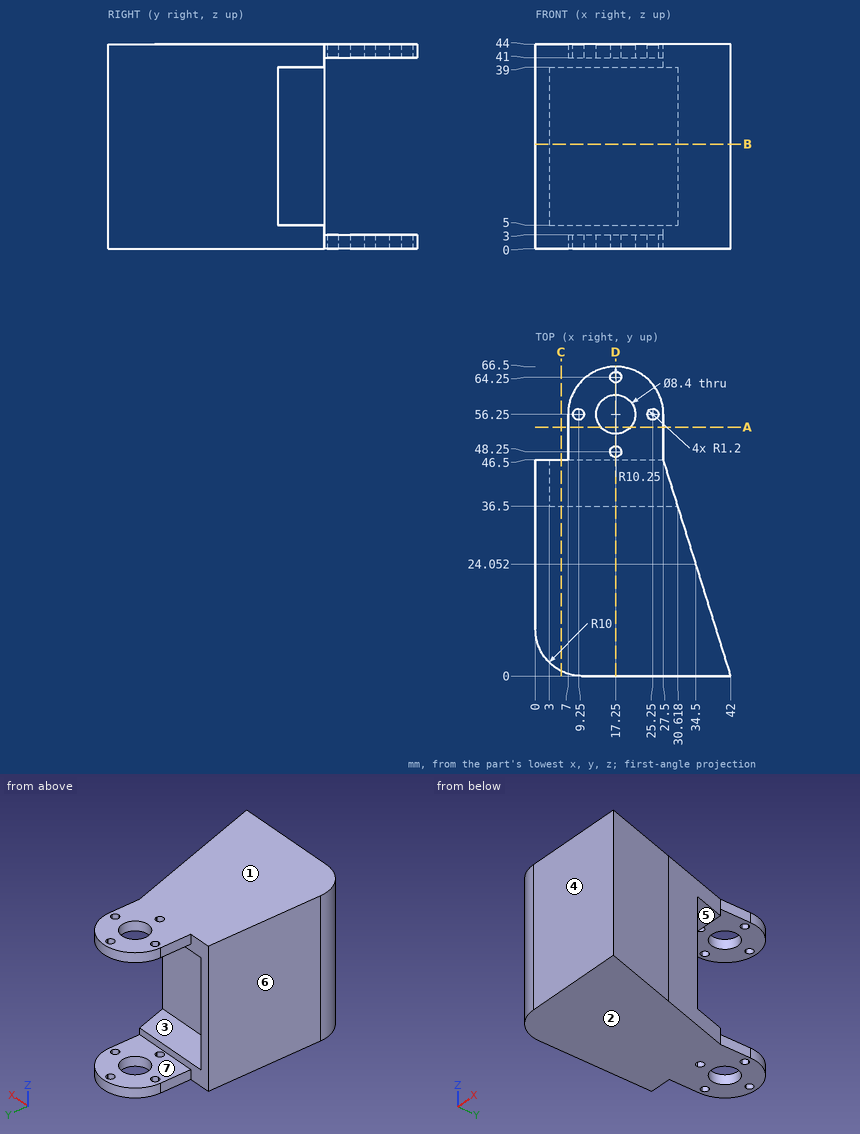
Verification items for this drawing (mm, ordinates from the low corner). A direction names the side the tool comes from. Give positions to 0.01 mm unless a question says otherwise; leave off trailing zeros. Order: outer loops, then holes, each group sorted by start corner. A loop starts at its lowest first (then second) coordinate and runs counter-clockwise, first axis right, second up.
1) Draft check along Z on the marked faces 1, 2, 3 and 4. Enter one of: released by +Z, released by -Z, zero draft, split by the parting line, or undercut.
Results are:
face 1: released by +Z
face 2: released by -Z
face 3: undercut
face 4: zero draft
2) Material ranges on probe 1 along Y at (x, z) = (17.25, 2.3); probe 2 along Z at (x, y) = (24, 38.5); probe 3 along X at (y, z) = (56, 42), recorded low to high.
Results are:
probe 1: y = 0 to 47.05, 49.45 to 52.05, 60.45 to 63.05, 65.45 to 66.5
probe 2: z = 0 to 5, 39 to 44
probe 3: x = 7 to 8.08, 10.42 to 13.06, 21.44 to 24.08, 26.42 to 27.5
3) Cross-section at B-B (z = 22.5). Record the boundary of the cut face in (x, y).
Results are:
outline: (0, 10) arc R10 ccw to (10, 0) - (42, 0) - (30.62, 36.5) - (3, 36.5) - (3, 46.5) - (0, 46.5) - close
4) Tool access check on the marked faces 5, 6 and 7. Record the directions out of +Z, -Z, +X, -X, +Y, -Y that give a thin tool (end or side, any length) a straight path to the whole face; none if there is none.
Results are:
face 5: +X, +Y
face 6: +Z, -Z, -X, +Y, -Y
face 7: +X, -X, +Y
5) Cross-section at C-C (x = 5.5). Record the boundary of the cut face in (y, z).
Results are:
outline: (1.07, 0) - (46.5, 0) - (46.5, 5) - (36.5, 5) - (36.5, 39) - (46.5, 39) - (46.5, 44) - (1.07, 44) - close
6) Cross-section at D-D (x = 17.25). Give the number of separate pieces and of enclosed holes in the cut face, then the cut area to 3 significant figures.
Results are:
separate pieces: 7
enclosed holes: 0
area: 1,750 mm2
7) Gauge pin test, flat ends, axial feed: pin 1 (10 mm diameter, centred on x = 17.5, y = 56, fed in from -Z); pin 2 (8 mm diameter, centred on y = 41.5, z = 31, fed in from +X); pin 3 (3.5 mm diameter, centred on y = 51.5, z = 42.5, fed in from +X); pin 4 (0.9 mm diameter, centred on y = 53.5, z = 1.5, fed in from -X). Record the tip position at first contact, or that the pin passes through.
Results are:
pin 1: stops at z = 0
pin 2: stops at x = 3
pin 3: stops at x = 27.5
pin 4: stops at x = 7
8) Cross-section at A-A (y = 53.5). Record the boundary of the cut face in (x, z) (1 decimal).
Results are:
outline: (7, 0) - (14.1, 0) - (14.1, 3) - (7, 3) - close; (7, 41) - (14.1, 41) - (14.1, 44) - (7, 44) - close; (20.4, 0) - (27.5, 0) - (27.5, 3) - (20.4, 3) - close; (20.4, 41) - (27.5, 41) - (27.5, 44) - (20.4, 44) - close
